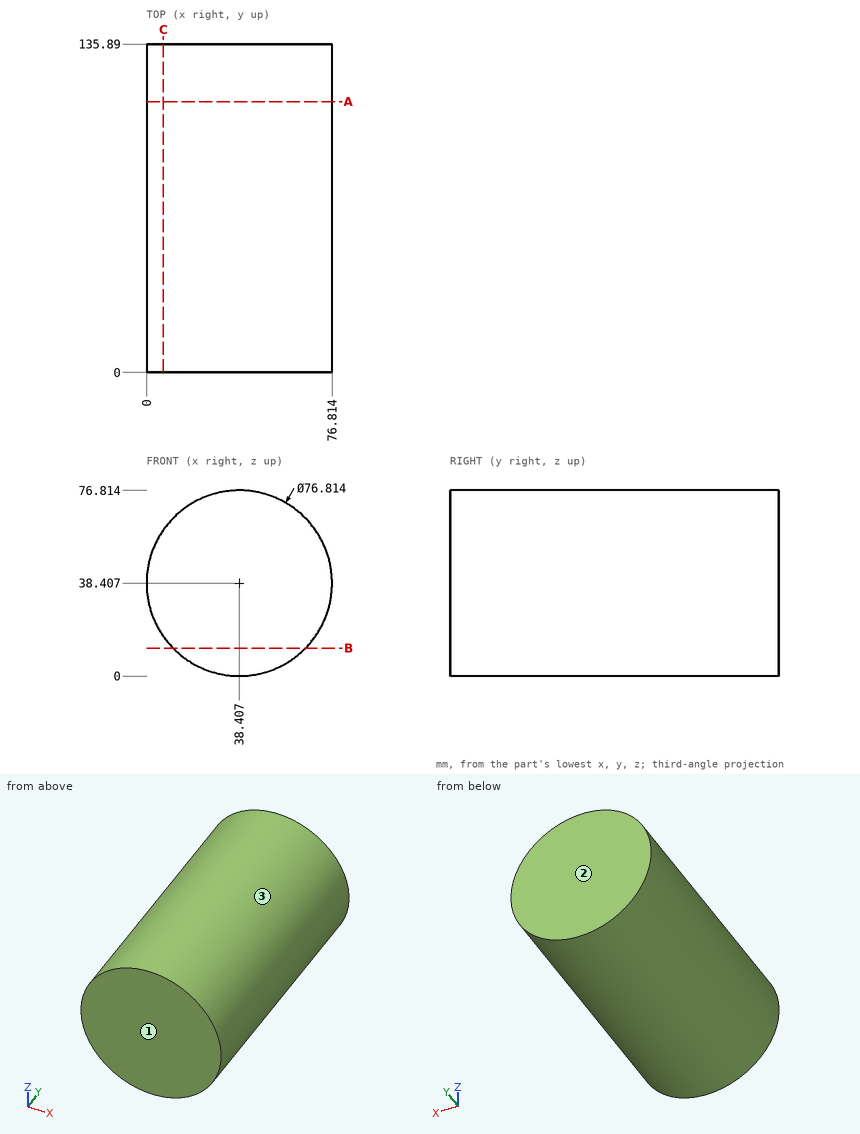
Design review of the part shown in the three views and the two pictorial views. Dimensions are in mm from the part's minimum x, y and z. Coordinates: 2 decimals unless noted, no trailing zeros. Loops run counter-clockwise (first coordinate to the right, second up) from the corner with the lowest first, then second, coordinate; pieces in that order, holes last.
Q1. We need section A-A on y = 112. State the section outline as (x, z) points.
Reported:
outline: circle Ø76.81 at (38.41, 38.41)
Q2. The part is to be moulded in two halves that separate along Y. For the marked faces 1, 2 and 3, say which applies: +Y half, -Y half, draft (parallel to the pull), parting line (faces both ways), or undercut.
Reported:
face 1: -Y half
face 2: +Y half
face 3: draft
Q3. We need section B-B on z = 11.5. State the section outline as (x, y) points, and give its area (3 significant figures).
Reported:
outline: (11, 0) - (65.81, 0) - (65.81, 135.89) - (11, 135.89) - close
area: 7,450 mm2
Q4. We need section C-C on x = 7. State the section outline as (y, z) points.
Reported:
outline: (0, 16.3) - (135.89, 16.3) - (135.89, 60.51) - (0, 60.51) - close
Q5. To check wall thickness, follow line 1 (Z direction, x = 38.5, y = 46.5); line 2 (X direction, y = 92, z = 12) (1 decimal); line 3 (X direction, y = 18.5, z = 31). State the ranges of each line that lie inside material, in increasing order.
Reported:
line 1: z = 0 to 76.81
line 2: x = 10.5 to 66.3
line 3: x = 0.72 to 76.09
Q6. For pin 1 (4 mm diameter, centred on x = 25.5, y = 119.5, fed in from +Z); pin 2 (1 mm diameter, centred on y = 18.5, z = 43, fed in from +X) (3 decimals); pin 3 (1.5 mm diameter, centred on x = 58, y = 109, fed in from -Z), all flat-tipped, find the tip position at first contact; note any pin that passes through.
Reported:
pin 1: stops at z = 75.23
pin 2: stops at x = 76.595
pin 3: stops at z = 4.94
